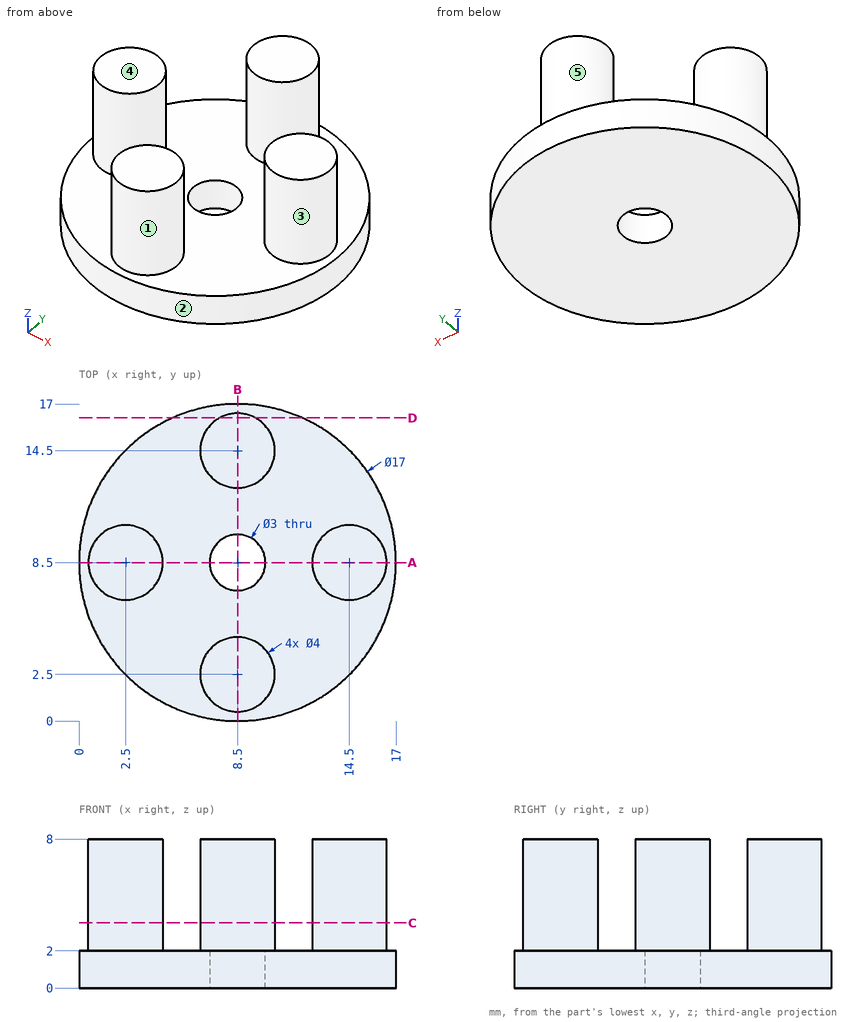
The drawing under review shows one solid part. Ordinate dimensions are in mm from its lowest x, y, z. A direction names the side the tool comes from. Round coordinates to 2 decimals unless told otherwise and drop trailing zeros. Write each loop counter-clockwise with the first axis right and the second up, starting at its lowest first coordinate (ties: lowest second). Pieces come first, ordered by that corner, then holes. Notation, with made-up numbers: (-18.75, 71) - (3.25, 71) arc R15 ccw to (3.25, 84) - close; hole circle Ø8 at (18, 85.25). An arc over 180 degrees is marked (long way). One line per question, with ' | ' between items.
Item 1: To check wall thickness, follow probe 1 along Y at (x, z) = (8.5, 1.1); probe 2 along Z at (x, y) = (2.5, 4.75); probe 3 along X at (y, z) = (2.5, 0.75). State the ranges of each line that lie inside material, in increasing order.
Resolved:
probe 1: y = 0 to 7, 10 to 17 | probe 2: z = 0 to 2 | probe 3: x = 2.48 to 14.52
Item 2: The part is to be moulded in two halves that separate along Y. For the marked faces 3, 4 and 5, say which applies: pulls with the +Y half, pulls with the -Y half, needs draft (parallel to the pull), parting line crosses it, or undercut.
Resolved:
face 3: parting line crosses it | face 4: needs draft | face 5: undercut
Item 3: Add section D-D, the plane y = 16.25. Give the boundary of the cut face in (x, z), then the cut area to 3 significant figures.
Resolved:
outline: (5.01, 0) - (11.99, 0) - (11.99, 2) - (9.47, 2) - (9.47, 8) - (7.53, 8) - (7.53, 2) - (5.01, 2) - close | area: 25.6 mm2
Item 4: For P1, Ø8, axis at x = 14.5, y = 6.5, coming from the -Z side; P2, Ø1.5, axis at y = 15, z = 5.5, coming from the -X side, all flat-tipped, find the tip position at first contact; note any pin that passes through.
Resolved:
P1: stops at z = 0 | P2: stops at x = 6.5
Item 5: For the marked faces 1 and 2, list the 3-axis set-ups (+Z, -Z, +X, -X, +Y, -Y) from which the entire face can be reached by the end or side of a thin tool; tool diameter is ignored.
Resolved:
face 1: +Z | face 2: +Z, -Z
Item 6: Add section A-A, the plane y = 8.5. Give the boundary of the cut face in (x, z).
Resolved:
outline: (0, 0) - (7, 0) - (7, 2) - (4.5, 2) - (4.5, 8) - (0.5, 8) - (0.5, 2) - (0, 2) - close; (10, 0) - (17, 0) - (17, 2) - (16.5, 2) - (16.5, 8) - (12.5, 8) - (12.5, 2) - (10, 2) - close
Item 7: Add section C-C, the plane z = 3.5. Give the boundary of the cut face in (x, y), then the cut area to 3 significant figures.
Resolved:
outline: circle Ø4 at (2.5, 8.5); circle Ø4 at (8.5, 2.5); circle Ø4 at (8.5, 14.5); circle Ø4 at (14.5, 8.5) | area: 50.3 mm2
